Work out the finished part from the listing and answer in its coordinate system (mm). Face numbers are marked on the shaded views. Coordinates: 2 decimals unless noted, no trailing zeros. Loops run counter-clockwise (first coordinate to the right, second up) from the corner with the lowest first, then second, coordinate; pieces in that order, holes last. Notation, with made-up numbers: (-19.75, -33) -> (-9.75, -33) arc R26 ccw to (-9.75, -10) -> close; hole circle Ø4 at (29.5, 88). An arc over 180 degrees is marked (long way). Use a Markdown table: item, result.
from build123d import *

# Parameters (mm, degrees)
F1_DEPTH = 4
F2_R     = 2
F2_R_2   = 3.5
F3_DEPTH = 25
F4_R     = 4.99999


# Not quite as in the source:
# - a fillet or chamfer is up to 0.001 mm smaller than in the source, because OpenCascade refuses the exact size


with BuildPart() as f1:
    # F0 (on Top) → F1 (new body)
    with BuildSketch(Plane.XY):
        Polygon((-5, 0), (-30, 0), (-30, -14), (30, -14), (30, 0), (5, 0), (5, 50), (-5, 50), align=None)
    extrude(amount=F1_DEPTH)

    # F2 (on face) → F3 (cut)
    with BuildSketch(Plane.XY.offset(4)):
        with Locations((-23.3714003116, -7)):
            Circle(F2_R)
        with Locations((20.7536797971, -7)):
            Circle(F2_R)
        with Locations((0, -7)):
            Circle(F2_R_2)
        with Locations((0, 46)):
            Circle(F2_R)
    extrude(amount=-F3_DEPTH, mode=Mode.SUBTRACT)

    # F4 (radius 5 in the source; OpenCascade refuses exactly that, so slightly less here)
    f4_edges = [f1.edges().sort_by_distance(p)[0] for p in [
        (-5, 50, 2),
        (5, 50, 2),
        (30, 0, 2),
        (30, -14, 2),
        (-30, -14, 2),
        (-30, 0, 2),
    ]]
    fillet(f4_edges, radius=F4_R)


solid = f1.part
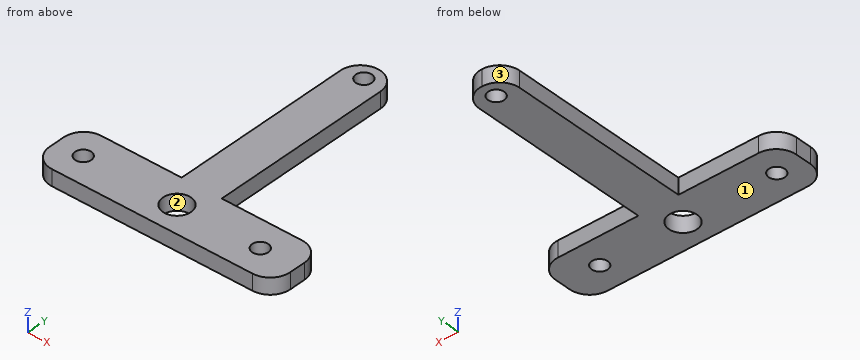
Q1. Section B-B on z = 2.9 is taken. State how many separate pieces and enclosed holes the cut face has, and give its area (3 significant figures).
Solved:
| item | result |
|---|---|
| separate pieces | 1 |
| enclosed holes | 4 |
| area | 1,230 mm² |
Q2. Section C-C on x = 21.5 is taken. Determine the outline of the cut face in (y, z).
Solved:
| item | result |
|---|---|
| outline | (-14, 0) -> (-8.86, 0) -> (-8.86, 4) -> (-14, 4) -> close; (-5.14, 0) -> (0, 0) -> (0, 4) -> (-5.14, 4) -> close |
Q3. Given pin 1 Ø2 at (y, z) = (16, 1.5) entering from -X; pin 2 Ø1.2 at (y, z) = (31, 2.5) entering from +X, each flat-ended and moving along its own axis, determine where each tip first touches the part or whether it passes through.
Solved:
| item | result |
|---|---|
| pin 1 | x = -5 |
| pin 2 | x = 5 |
Q4. Section D-D on y = 46 is taken. Determine the outline of the cut face in (x, z), and give its area (3 significant figures).
Solved:
| item | result |
|---|---|
| outline | (-4.9, 0) -> (-2, 0) -> (-2, 4) -> (-4.9, 4) -> close; (2, 0) -> (4.9, 0) -> (4.9, 4) -> (2, 4) -> close |
| area | 23.2 mm² |
Q5. Determine the mould class of the marked faces 1, 2 and 3 for opening direction X: pulls with the +X half, pulls with the -X half, needs draft (parallel to the pull), parting line crosses it, or undercut.
Solved:
| item | result |
|---|---|
| face 1 | needs draft |
| face 2 | undercut |
| face 3 | pulls with the -X half |
Q6. Section A-A on y = -7 is taken. Determine the outline of the cut face in (x, z), and give its area (3 significant figures).
Solved:
| item | result |
|---|---|
| outline | (-30, 0) -> (-25.37, 0) -> (-25.37, 4) -> (-30, 4) -> close; (-21.37, 0) -> (-3.5, 0) -> (-3.5, 4) -> (-21.37, 4) -> close; (3.5, 0) -> (18.75, 0) -> (18.75, 4) -> (3.5, 4) -> close; (22.75, 0) -> (30, 0) -> (30, 4) -> (22.75, 4) -> close |
| area | 180 mm² |
Q7. Consider line 1 (Y direction, x = 0, z = 2.5); line 2 (Y direction, x = -10.5, z = 0.45); line 3 (X direction, y = 5, z = 1.25). Determine where each line is inside the solid, lowest interval first. Write a range as [from, to].
Solved:
| item | result |
|---|---|
| line 1 | [-14, -10.5], [-3.5, 44], [48, 50] |
| line 2 | [-14, 0] |
| line 3 | [-5, 5] |
